Design review of the part built by this model. Coordinates are the model's own, in mm. Give positions to 0.01 mm unless a question says otherwise; leave off trailing zeros. Write each loop counter-clockwise with the first axis right and the second up, starting at its lowest first coordinate (ties: lowest second). Pieces come first, ordered by that corner, then holes. Notation, with made-up numbers: (43, -4) -> (52, -4) arc R37 cw to (52, 35) -> close; hole circle Ø7 at (5, -7.5). An arc over 180 degrees is marked (long way). Return JSON: item names as keys, results as strings. Group by question number.
Autodesk Inventor part; units mm, degrees
ref_plane "YZ Plane" through (0, 0, 0) normal (1, 0, 0) x (0, 1, 0)
ref_plane "XZ Plane" through (0, 0, 0) normal (0, 1, 0) x (-1, 0, 0)
ref_plane "XY Plane" through (0, 0, 0) normal (0, 0, 1) x (1, 0, 0)
sketch "Boceto1" plane through (0, 0, 0) normal (0, 1, 0) x (-1, 0, 0)
  line L0 (-12.5, -12.5) -> (12.5, -12.5) construction
  line L1 (12.5, -12.5) -> (12.5, 12.5) construction
  line L2 (12.5, 12.5) -> (-12.5, 12.5) construction
  line L3 (-12.5, 12.5) -> (-12.5, -12.5) construction
  line L4 (-12.5, -12.5) -> (12.5, 12.5) construction
  line L5 (12.5, -12.5) -> (-12.5, 12.5) construction
  circle A0 centre (0, 0) radius 17.6777
  dimension "d0" = 25
  dimension "d1" = 25
extrude "Extrusión1" add sketch "Boceto1" along normal blind 5
sketch "Boceto2" plane through (0, 0, 0) normal (1, 0, 0) x (0, 1, 0)
  line L0 (5, -17.6777) -> (5, 17.6777) construction
  line L1 (5, 0) -> (30, 0)
  line L2 (30, 0) -> (5, 17.6777)
  line L3 (20, 0) -> (20, 7.0711)
  line L4 (5, 0) -> (5, 17.6777)
  line L5 (-6, 0) -> (36, 0)
  point P0 (0, 0)
  dimension "d4" = 25
  dimension "d5" = 15
revolve "Revolución1" add sketch "Boceto2" angle 360 about axis through (0, -10, 0) along (0, 1, 0) contours L4 L2 L3 L1
sketch "Boceto3" plane through (0, 20, 0) normal (0, 1, 0) x (1, 0, 0)
  point P0 (0, 0)
  point P1 (0, 0)
hole "Agujero1" at (0, 20, 0) direction (0, -1, 0) diameter 3.6 end through all
sketch "Boceto4" plane through (0, 0, 0) normal (0, -1, 0) x (1, 0, 0)
  point P0 (0, 0)
chamfer "Chaflán1" distance 4 angle 45 1 edges at (0, 0, -1.8)
chamfer "Chaflán2" distance 1 angle 45 2 edges at (17.6777, 0, 0) (0, 20, -7.0711)
chamfer "Chaflán3" distance 1 angle 45 1 edges at (0, 20, -1.8)
properties part number "PesaGrua"
Q1. Take a section at B-B, the plane x = 0. Give the boundary of the cut face in (y, z), plus the area to 3 significant figures.
Q2. Take a section at A-A, the plane z = 0. Give the boundary of the cut face in (x, y), plus the area to 3 significant figures.
Q3. Mouldability with a two-part tool opening along Z and no side actions: class faces 1 (the face through (-7, 0, 0)), 2 (the face through (-6, 18, -6)), 3 (the face through (-0.541, 11.395, 1.717)), 4 (the face through (-0.616, 3.75, 1.956)) as +Z half, -Z half, draft (parallel to the pull), parting line (faces both ways), or undercut.
Q4. Insertion check: pin 1 (10 mm diameter, centred on y = 4.5, z = -12.5, fed in from +X); pin 2 (12 mm diameter, centred on x = -10, y = 16.5, fed in from -Z); pin 3 (6 mm diameter, centred on x = 0, z = 0, fed in from -Y). Each pin has a flat end and moves straight along its axis. Give the tip position at first contact, or say it passes through.
Q5. Take a section at C-C, the plane y = 15.25. Give the boundary of the cut face in (x, z).
Q6. For L1, parallel to X at y = 14, z = 0; L2, parallel to X at y = 8.5, z = 0; L3, parallel to Z at x = 0, y = 7.5, list the stretches that pass through material, from the lowest coordinate up. Write a range as from..to.
Q7. Take a section at D-D, the plane y = 18.5. Give the boundary of the cut face in (x, z), plus the area to 3 significant figures.
Final values:
{
 "1": {"outline": "(0, -16.68) -> (1, -17.68) -> (5, -17.68) -> (19.18, -7.65) -> (20, -6.07) -> (20, -2.8) -> (19, -1.8) -> (4, -1.8) -> (0, -5.8) -> close; (0, 5.8) -> (4, 1.8) -> (19, 1.8) -> (20, 2.8) -> (20, 6.07) -> (19.18, 7.65) -> (5, 17.68) -> (1, 17.68) -> (0, 16.68) -> close", "area": "457 mm²"},
 "2": {"outline": "(-17.68, 1) -> (-16.68, 0) -> (-5.8, 0) -> (-1.8, 4) -> (-1.8, 19) -> (-2.8, 20) -> (-6.07, 20) -> (-7.65, 19.18) -> (-17.68, 5) -> close; (1.8, 4) -> (5.8, 0) -> (16.68, 0) -> (17.68, 1) -> (17.68, 5) -> (7.65, 19.18) -> (6.07, 20) -> (2.8, 20) -> (1.8, 19) -> close", "area": "457 mm²"},
 "3": {"face 1": "draft", "face 2": "parting line", "face 3": "undercut", "face 4": "undercut"},
 "4": {"pin 1": "stops at x = 16.01", "pin 2": "stops at z = -11.25", "pin 3": "stops at y = 2.8"},
 "5": {"outline": "circle Ø20.86 at (0, 0); hole circle Ø3.6 at (0, 0)"},
 "6": {"L1": "x = -11.31..-1.8, 1.8..11.31", "L2": "x = -15.2..-1.8, 1.8..15.2", "L3": "z = -15.91..-1.8, 1.8..15.91"},
 "7": {"outline": "circle Ø16.26 at (0, 0); hole circle Ø3.6 at (0, 0)", "area": "198 mm²"}
}
